```python
from build123d import *

# Parameters (mm, degrees)
BOSS_EXTRUDE2_DEPTH     = 18
CUT_EXTRUDE1_START      = -10
CUT_EXTRUDE1_DEPTH      = 10
SKETCH4_R               = 4.577705579
CUT_EXTRUDE2_DEPTH      = 52.544224249
CUT_EXTRUDE3_DEPTH      = 52.544224249
SKETCH6_R               = 3
CUT_EXTRUDE4_DEPTH      = 10
CUT_EXTRUDE5_REACH      = 52.723
CUT_EXTRUDE5_END_RADIUS = 19
SKETCH7_R               = 1.5


# Read off the part's stored shape, not the designer's step: Cut-Extrude1
with BuildPart() as part:
    # Sketch1 → Boss-Extrude2 (new, symmetric)
    with BuildSketch(Plane.XY):
        with BuildLine():
            Line((18.027756377, -13), (21.997756377, -13))
            Line((21.997756377, -13), (21.997756377, -1))
            Line((21.997756377, -1), (42.997756377, -1))
            Line((42.997756377, -1), (42.997756377, 9))
            Line((42.997756377, 9), (22.627416998, 9))
            ThreePointArc((22.627416998, 9), (0, 17), (-22.627416998, 9))
            Line((-22.627416998, 9), (-42.997756377, 9))
            Line((-42.997756377, 9), (-42.997756377, -1))
            Line((-42.997756377, -1), (-21.997756377, -1))
            Line((-21.997756377, -1), (-21.997756377, -13))
            Line((-21.997756377, -13), (-18.027756377, -13))
            ThreePointArc((-18.027756377, -13), (0, 0), (18.027756377, -13))
        make_face()
    extrude(amount=BOSS_EXTRUDE2_DEPTH, both=True)

    # Cut-Extrude1 outline → Cut-Extrude1 (cut)
    with BuildSketch(Plane(origin=(0, 9, 0), x_dir=(1, 0, 0), z_dir=(0, 1, 0)).offset(CUT_EXTRUDE1_START)):
        with BuildLine():
            ThreePointArc((42.997756377, 0), (41.998910053, -9.214044053), (39.048777874, -18))
            Line((39.048777874, -18), (42.997756377, -18))
            Line((42.997756377, -18), (42.997756377, 0))
        make_face()
        with BuildLine():
            ThreePointArc((39.048777874, 18), (41.998910053, 9.214044053), (42.997756377, 0))
            Line((42.997756377, 0), (42.997756377, 18))
            Line((42.997756377, 18), (39.048777874, 18))
        make_face()
        with BuildLine():
            Line((-42.997756377, -18), (-39.048777874, -18))
            ThreePointArc((-39.048777874, -18), (-41.998910053, -9.214044053), (-42.997756377, 0))
            Line((-42.997756377, 0), (-42.997756377, -18))
        make_face()
        with BuildLine():
            Line((-42.997756377, 18), (-42.997756377, 0))
            ThreePointArc((-42.997756377, 0), (-41.998910053, 9.214044053), (-39.048777874, 18))
            Line((-39.048777874, 18), (-42.997756377, 18))
        make_face()
    extrude(amount=CUT_EXTRUDE1_DEPTH, mode=Mode.SUBTRACT)

    # Sketch4 → Cut-Extrude2 (cut, through all)
    with BuildSketch(Plane(origin=(0, 9, 0), x_dir=(1, 0, 0), z_dir=(0, 1, 0))):
        with Locations(Location((-31, 0, 0), (0, 0, 180))):
            Circle(SKETCH4_R)
        with Locations(Location((31, 0, 0), (0, 0, 270))):
            Circle(SKETCH4_R)
    extrude(amount=-CUT_EXTRUDE2_DEPTH, mode=Mode.SUBTRACT)

    # Sketch5 → Cut-Extrude3 (cut, through all)
    with BuildSketch(Plane(origin=(0, 9, 0), x_dir=(1, 0, 0), z_dir=(0, 1, 0))):
        with BuildLine():
            Line((-22.627416998, 8.593370233), (-22.627416998, -8.593370233))
            ThreePointArc((-22.627416998, -8.593370233), (-19.002243623, 0), (-22.627416998, 8.593370233))
        make_face()
        with BuildLine():
            Line((22.627416998, 8.593370233), (22.627416998, -8.593370233))
            ThreePointArc((22.627416998, -8.593370233), (19.002243623, 0), (22.627416998, 8.593370233))
        make_face()
    extrude(amount=CUT_EXTRUDE3_DEPTH, mode=Mode.SUBTRACT)

    # Sketch6 → Cut-Extrude4 (cut)
    with BuildSketch(Plane(origin=(0, 17, 0), x_dir=(1, 0, 0), z_dir=(0, 1, 0))):
        with Locations(Location((0, 0, 0), (0, 0, 270))):
            Circle(SKETCH6_R)
    extrude(amount=-CUT_EXTRUDE4_DEPTH, mode=Mode.SUBTRACT)

    # Cut-Extrude5: up to this cylinder (the profile starts outside it)
    cut_extrude5_end = Plane(origin=(0, -19, 0), z_dir=(0, 0, -1)) * Cylinder(CUT_EXTRUDE5_END_RADIUS, 144.446, mode=Mode.PRIVATE)
    # Sketch7 → Cut-Extrude5 (cut, up to the surface)
    with BuildSketch(Plane(origin=(0, 7, 0), x_dir=(1, 0, 0), z_dir=(0, 1, 0)), mode=Mode.PRIVATE) as cut_extrude5_sk1:
        with Locations(Location((0, 0, 0), (0, 0, 270))):
            Circle(SKETCH7_R)
    cut_extrude5_tool1 = extrude(cut_extrude5_sk1.sketch, amount=-CUT_EXTRUDE5_REACH, mode=Mode.PRIVATE) - cut_extrude5_end
    add(cut_extrude5_tool1.solids().sort_by_distance((0, 7, 0))[0], mode=Mode.SUBTRACT)


solid = part.part
```
Check sheet for the modelled part. Datum: model origin and axes. Units: mm. A direction names the side the tool comes from. Round coordinates to 2 decimals unless told otherwise and drop trailing zeros. Order: outer loops, then holes, each group sorted by start corner. A loop starts at its lowest first (then second) coordinate and runs counter-clockwise, first axis right, second up. Notation, with made-up numbers: (66.25, 82.25) -> (94.25, 82.25) arc R31 ccw to (94.25, 113.25) -> close; hole circle Ø3 at (-8.5, -33.75). An arc over 180 degrees is marked (long way). Use CSV: the item, a comma, the result in double quotes.
(1) Draft check along Z on faces 5 (the face through (0.45, 3.52, 1.43)), 6 (the face through (-1, 6, 18)), 7 (the face through (21.998, -7, 0)), 8 (the face through (26.939, 4.07, 2.112)). Enter one of: pulls with the +Z half, pulls with the -Z half, needs draft (parallel to the pull), parting line crosses it, or undercut.
Worked out:
face 5,"undercut"
face 6,"pulls with the +Z half"
face 7,"needs draft"
face 8,"undercut"
(2) Tool access check on faces 1 (the face through (-19.003, 9.984, 0.134)), 2 (the face through (0.9, 12.07, 2.86)), 3 (the face through (35, -1, -4)), 4 (the face through (19.003, 9.984, 0.134)). Record the directions out of +Z, -Z, +X, -X, +Y, -Y that give a thin tool (end or side, any length) a straight path to the whole face; none if there is none.
Worked out:
face 1,"-X, +Y"
face 2,"+Y"
face 3,"+Z, -Z, +X, -Y"
face 4,"+X, +Y"
(3) Cross-section at B-B (y = -5.5). Record the boundary of the cut face in (x, z).
Worked out:
outline,"(-22, -18) -> (-13.37, -18) -> (-13.37, 18) -> (-22, 18) -> close; (13.37, -18) -> (22, -18) -> (22, 18) -> (13.37, 18) -> close"
(4) Cross-section at A-A (x = 31). Record the boundary of the cut face in (y, z), and give its area (3 significant figures).
Worked out:
outline,"(-1, -18) -> (9, -18) -> (9, -4.58) -> (-1, -4.58) -> close; (-1, 4.58) -> (9, 4.58) -> (9, 18) -> (-1, 18) -> close"
area,"268 mm²"
(5) Cross-section at D-D (x = 0). Record the boundary of the cut face in (y, z), and give its area (3 significant figures).
Worked out:
outline,"(0, -18) -> (17, -18) -> (17, -3) -> (7, -3) -> (7, -1.5) -> (0, -1.5) -> close; (0, 1.5) -> (7, 1.5) -> (7, 3) -> (17, 3) -> (17, 18) -> (0, 18) -> close"
area,"531 mm²"
(6) Material ranges on line 1 along Z through (x, y) = (-31, 5.75); line 2 along X through (y, z) = (10.5, 0); line 3 along Y through (x, z) = (28.5, 6), recorded low to high. Write a range as from..to.
Worked out:
line 1,"-18..-4.58, 4.58..18"
line 2,"-19..-3, 3..19"
line 3,"-1..9"
(7) Depth check by flat-ended pin: pin 1 (2 mm diameter, centred on y = 4.5, z = -5, fed in from +X); pin 2 (8 mm diameter, centred on x = -31.5, z = -3.5, fed in from +Y); pin 3 (6 mm diameter, centred on x = 7.5, z = -3, fed in from -Y). Enter the tip coordinate at first touch or a pass-through.
Worked out:
pin 1,"x = 42.81"
pin 2,"y = 9"
pin 3,"y = -3.16"
(8) Cross-section at C-C (y = 2). Record the boundary of the cut face in (x, z), and give its area (3 significant figures).
Worked out:
outline,"(-39.05, -18) -> (39.05, -18) arc R43 ccw to (39.05, 18) -> (-39.05, 18) arc R43 ccw to start; hole circle Ø9.16 at (-31, 0); hole circle Ø3 at (0, 0); hole circle Ø9.16 at (31, 0)"
area,"2,860 mm²"
